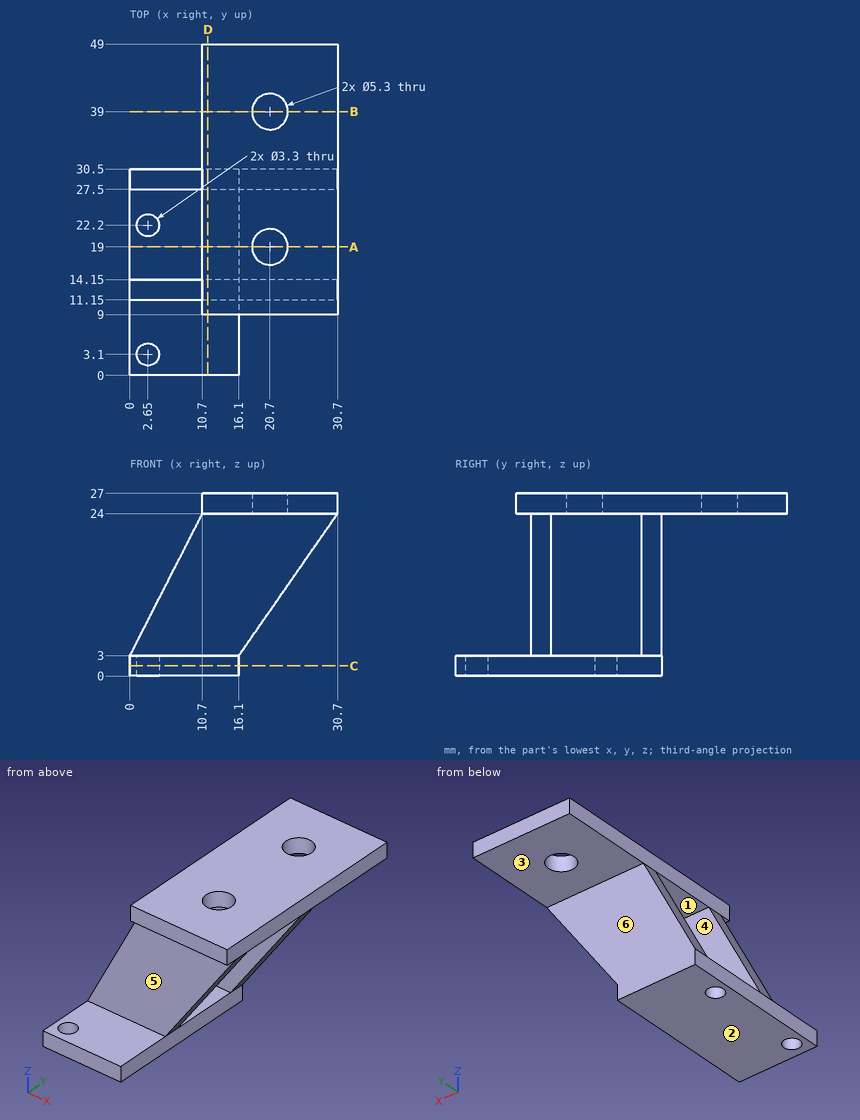
Verification items for this drawing (mm, ordinates from the low corner). A direction names the side the tool comes from. Give positions to 0.01 mm unless a question says otherwise; leave off trailing zeros. Loops run counter-clockwise (first coordinate to the right, second up) from the corner with the lowest first, then second, coordinate; pieces in that order, holes last. Notation, with made-up numbers: M 74.25,65 L 79.25,65 A29 cw 79.25,97 Z; hole C 56.25,1 d7. An arc over 180 degrees is marked long. Write item = value, one per line. Start each with the question number.
1. Section check C-C, the plane z = 1.5. Enter the section's corners in (x, y), plus the area to 3 significant figures.
2. Tool access check on the marked faces 1, 2 and 3. Record the directions out of +Z, -Z, +X, -X, +Y, -Y that give a thin tool (end or side, any length) a straight path to the whole face; none if there is none.
3. Section check D-D, the plane x = 11.5. Enter the section's corners in (y, z), plus the area to 4 significant figures.
4. Go/stop test with flat-tipped pins: P1, Ø1.5, axis at y = 23.5, z = 25, coming from the -X side; P2, Ø2, axis at x = 21.5, z = 11.5, coming from the +Y side; P3, Ø5, axis at y = 18, z = 13, coming from the +X side; P4, Ø1, axis at x = 14, z = 19.5, coming from the -Y side. Record where each tip stops, or that it passes through.
5. Section check B-B, the plane y = 39. Enter the section's corners in (x, z).
6. Thickness scan on probe 1 along Y at (x, z) = (20.7, 25.35); probe 2 along Y at (x, z) = (2.65, 0.95); probe 3 along Y at (x, z) = (6.5, 14.25). Record the ranges inside material, lowest first.
7. Draft check along Y on the marked faces 4, 5 and 6. Enter one of: +Y half, -Y half, draft (parallel to the pull), parting line (faces both ways), or undercut.
8. Section check A-A, the plane y = 19. Enter the section's corners in (x, z).
Values follow:
q1.outline = M 0,0 L 16.1,0 L 16.1,30.5 L 0,30.5 Z; hole C 2.65,3.1 d3.3; hole C 2.65,22.2 d3.3
q1.area = 474 mm^2
q2.face_1 = +X, -X
q2.face_2 = -Z, +X, -X, +Y, -Y
q2.face_3 = -Z, +X, -X, +Y
q3.outline = M 0,0 L 30.5,0 L 30.5,24 L 49,24 L 49,27 L 9,27 L 9,24 L 11.15,24 L 11.15,3 L 0,3 Z; hole M 14.15,3 L 27.5,3 L 27.5,24 L 14.15,24 Z
q3.area = 337.5 mm^2
q4.P1 = 10.7
q4.P2 = 30.5
q4.P3 = through
q4.P4 = 11.15
q5.outline = M 10.7,24 L 18.05,24 L 18.05,27 L 10.7,27 Z; M 23.35,24 L 30.7,24 L 30.7,27 L 23.35,27 Z
q6.probe_1 = 9 to 16.35, 21.65 to 36.35, 41.65 to 49
q6.probe_2 = 0 to 1.45, 4.75 to 20.55, 23.85 to 30.5
q6.probe_3 = 11.15 to 14.15, 27.5 to 30.5
q7.face_4 = undercut
q7.face_5 = -Y half
q7.face_6 = +Y half
q8.outline = M 0,0 L 16.1,0 L 16.1,3 L 0,3 Z; M 10.7,24 L 18.05,24 L 18.05,27 L 10.7,27 Z; M 23.35,24 L 30.7,24 L 30.7,27 L 23.35,27 Z
